```python
from build123d import *

# Parameters (mm, degrees)
SKETCH_R      = 13
SKETCH_R_2    = 10
PAD_DEPTH     = 6
SKETCH001_R   = 13
SKETCH001_R_2 = 8.5
PAD001_DEPTH  = 20
SKETCH002_R   = 13
PAD002_DEPTH  = 3
SKETCH003_R   = 2.5
POCKET_DEPTH  = 29.001
CHAMFER_SIZE  = 0.5


with BuildPart() as part:
    # Sketch → Pad (new body)
    with BuildSketch(Plane.XY):
        Circle(SKETCH_R)
        Circle(SKETCH_R_2, mode=Mode.SUBTRACT)
    extrude(amount=PAD_DEPTH)

    # Sketch001 (on Face4 of Pad) → Pad001 (join)
    with BuildSketch(Plane.XY.offset(6)):
        Circle(SKETCH001_R)
        Circle(SKETCH001_R_2, mode=Mode.SUBTRACT)
    extrude(amount=PAD001_DEPTH)

    # Sketch002 (on Face5 of Pad001) → Pad002 (join)
    with BuildSketch(Plane.XY.offset(26)):
        Circle(SKETCH002_R)
    extrude(amount=PAD002_DEPTH)

    # Sketch003 (on Face7 of Pad002) → Pocket (cut, through all)
    with BuildSketch(Plane.XY.offset(29)):
        Circle(SKETCH003_R)
    extrude(amount=-POCKET_DEPTH, mode=Mode.SUBTRACT)

    # Chamfer
    chamfer_edges = [part.edges().sort_by_distance(p)[0] for p in [
        (-10, 0, 0),
    ]]
    chamfer(chamfer_edges, length=CHAMFER_SIZE)


solid = part.part
```
Verification items for the finished model (mm, model axes). A direction names the side the tool comes from. Coordinates: 2 decimals unless noted, no trailing zeros. Order: outer loops, then holes, each group sorted by start corner. A loop starts at its lowest first (then second) coordinate and runs counter-clockwise, first axis right, second up. Notation, with made-up numbers: (43, -4) -> (58, -4) arc R21 ccw to (58, 4) -> close; hole circle Ø3 at (17, 36). An arc over 180 degrees is marked (long way). Put each result on its own line as item: value. Start each with the question number.
1) Release check for a two-part mould opening along X. For faces 3 (the cylindrical face through (-10.316, -7.91, 14.297)), 4 (the flat face through (-4.5, -7.4, 6)), 5 (the flat face through (-9, 6, 0)) record: pulls with the +X half, pulls with the -X half, needs draft (parallel to the pull), parting line crosses it, or undercut.
2) Go/stop test with flat-tipped pins: pin 1 (2 mm diameter, centred on x = 10, z = 6.5, fed in from +Y); pin 2 (13.5 mm diameter, centred on x = 3.5, y = -2.5, fed in from -Z); pin 3 (10 mm diameter, centred on x = 10.5, z = 13.5, fed in from -Y); pin 4 (3 mm diameter, centred on x = 0, y = 0, fed in from -Z). Record where each tip stops, or that it passes through.
3) Cross-section at A-A (y = 0). Enter the section's corners in (x, z).
4) Tool access check on faces 1 (the flat face through (2, -2, 26)), 2 (the cylindrical face through (-0.54, -2.44, 27.52)). Record the directions out of +Z, -Z, +X, -X, +Y, -Y that give a thin tool (end or side, any length) a straight path to the whole face; none if there is none.
5) Cross-section at C-C (z = 18.5). Enter the section's corners in (x, y).
6) Material ranges on L1, parallel to Y at x = 0.25, z = 9; L2, parallel to Y at x = 0, z = 26.9; L3, parallel to Z at x = 3.25, y = 3.5, recorded low to high.
Geometry check:
1. face 3: parting line crosses it
1. face 4: undercut
1. face 5: needs draft
2. pin 1: stops at y = 9.38
2. pin 2: stops at z = 0
2. pin 3: stops at y = -11.78
2. pin 4: passes through
3. outline: (-13, 0) -> (-10.5, 0) -> (-10, 0.5) -> (-10, 6) -> (-8.5, 6) -> (-8.5, 26) -> (-2.5, 26) -> (-2.5, 29) -> (-13, 29) -> close; (2.5, 26) -> (8.5, 26) -> (8.5, 6) -> (10, 6) -> (10, 0.5) -> (10.5, 0) -> (13, 0) -> (13, 29) -> (2.5, 29) -> close
4. face 1: -Z
4. face 2: +Z, -Z
5. outline: circle Ø26 at (0, 0); hole circle Ø17 at (0, 0)
6. L1: y = -13 to -8.5, 8.5 to 13
6. L2: y = -13 to -2.5, 2.5 to 13
6. L3: z = 26 to 29
